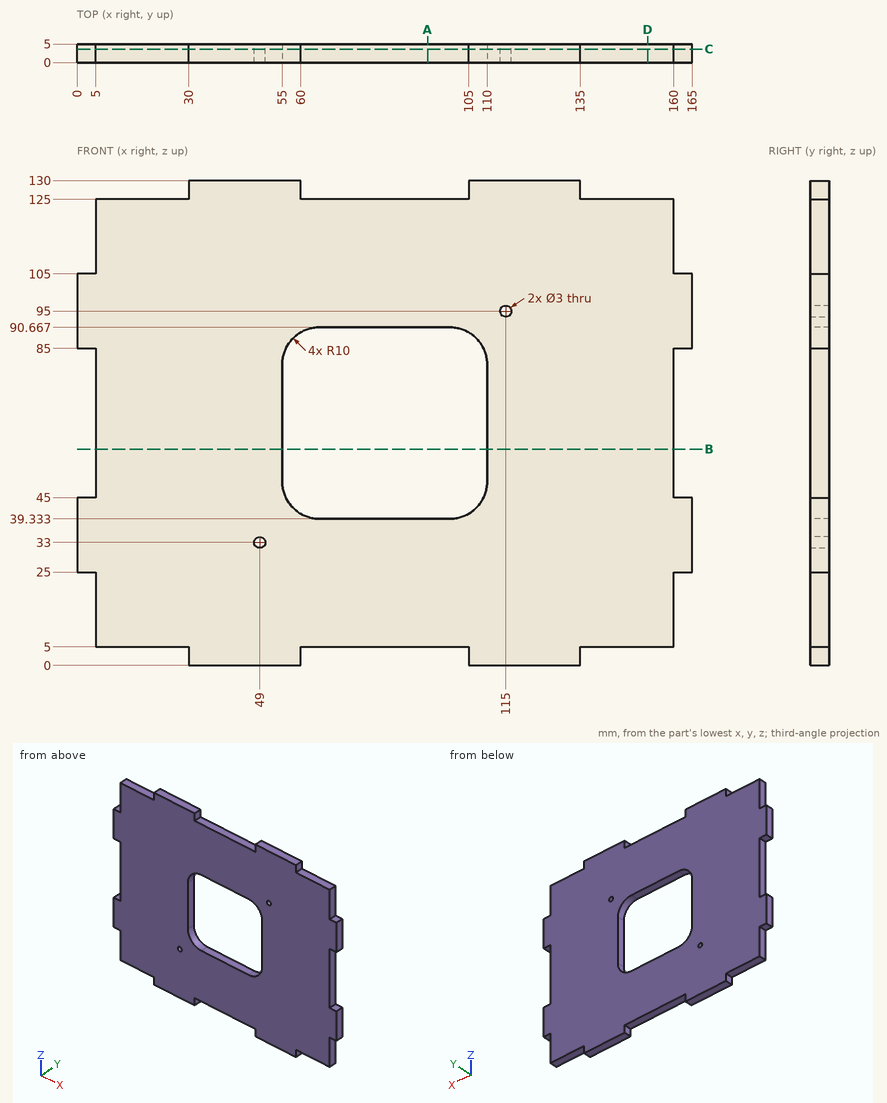
Source: three-view drawing plus pictorial views. Frame: mm from the lowest corner of the part. Give positions to 0.01 mm unless a question says otherwise; leave off trailing zeros. Order: outer loops, then holes, each group sorted by start corner. A loop starts at its lowest first (then second) coordinate and runs counter-clockwise, first axis right, second up. Notation, with made-up numbers: (56.5, -21) - (65.5, -21) arc R33 ccw to (65.5, 10) - close; hole circle Ø5 at (73, 29). An arc over 180 degrees is marked (long way). Answer as a JSON object with one key per item and string values. Group by question number.
Q1. Cut plane B-B, the plane z = 58. Output: boundary loops of the cut face in (x, y).
Q2. Cut plane D-D, the plane x = 153. Output: boundary loops of the cut face in (y, z).
Q3. First-contact query: pin 1 Ø1.5 at (y, z) = (1.5, 3) entering from -X; pin 2 Ø1.5 at (x, y) = (83, 2.5) entering from +Z; pin 3 Ø1.5 at (y, z) = (3.5, 3.5) entering from +X. Flat tips, straight axial feed; report the tip coordinate or a pass-through.
Q4. Cut plane C-C, the plane y = 3.65. Count the separate pieces of the cut face and the enclosed holes in it, then the cut area to 3 significant figures.
Q5. Cut plane A-A, the plane x = 94. Output: boundary loops of the cut face in (y, z), then the cut area to 3 significant figures.
Q6. Line query: probe 1 along X at (y, z) = (3.7, 49) (1 decimal); probe 2 along X at (y, z) = (1.9, 95); probe 3 along Z at (x, y) = (115, 1.65). Output: solid intervals per line, ascending.
Results:
{
 "1": {"outline": "(5, 0) - (55, 0) - (55, 5) - (5, 5) - close; (110, 0) - (160, 0) - (160, 5) - (110, 5) - close"},
 "2": {"outline": "(0, 5) - (5, 5) - (5, 125) - (0, 125) - close"},
 "3": {"pin 1": "x = 30", "pin 2": "z = 125", "pin 3": "x = 135"},
 "4": {"separate pieces": "1", "enclosed holes": "3", "area": "16,800 mm^2"},
 "5": {"outline": "(0, 5) - (5, 5) - (5, 39.33) - (0, 39.33) - close; (0, 90.67) - (5, 90.67) - (5, 125) - (0, 125) - close", "area": "343 mm^2"},
 "6": {"probe 1": "5 to 55, 110 to 160", "probe 2": "0 to 113.5, 116.5 to 165", "probe 3": "0 to 93.5, 96.5 to 130"}
}
